from build123d import *

# Parameters (mm, degrees)
PAD_DEPTH = 5


with BuildPart() as part:
    # Sketch → Pad (new body)
    with BuildSketch(Plane.XZ.offset(-65.300003)):
        with BuildLine():
            Line((62.415147, 3.02512), (62.415147, 5.02512))
            Line((62.415147, 5.02512), (55.415147, 5.02512))
            Line((55.415147, 5.02512), (55.415147, 3.02512))
            Line((55.415147, 3.02512), (54.415147, 3.02512))
            add(Edge.make_bspline(
                [(52.415147, 3.02512), (52.415147, 2.62512), (53.415147, 2.62512), (54.415147, 2.62512), (54.415147, 3.02512)],
                knots=[0, 0, 0, 1.570796, 1.570796, 3.141593, 3.141593, 3.141593], degree=2, weights=[1, 0.707107, 1, 0.707107, 1]))
            Line((52.415147, 3.02512), (49.415147, 3.02512))
            add(Edge.make_bspline(
                [(47.415156, 3.02512), (47.417952, 2.625118), (48.417947, 2.625118), (49.417943, 2.625118), (49.415147, 3.02512)],
                knots=[0.003328, 0.003328, 0.003328, 1.574124, 1.574124, 3.144921, 3.144921, 3.144921], degree=2, weights=[1, 0.707107, 1, 0.707107, 1]))
            Line((47.415156, 3.02512), (44.415156, 3.02512))
            add(Edge.make_bspline(
                [(42.415165, 3.02512), (42.417868, 2.625118), (43.417863, 2.625118), (44.417859, 2.625118), (44.415156, 3.02512)],
                knots=[0.003218, 0.003218, 0.003218, 1.574014, 1.574014, 3.14481, 3.14481, 3.14481], degree=2, weights=[1, 0.707107, 1, 0.707107, 1]))
            Line((42.415165, 3.02512), (40.460414, 4.579441))
            ThreePointArc((40.460414, 4.579441), (40.379979, 4.857522), (40.616008, 5.02512))
            Line((40.616008, 5.02512), (53.415147, 5.02512))
            add(Edge.make_bspline(
                [(64.915147, 5.02512), (59.165147, 9.713985), (53.415147, 5.02512)],
                knots=[0.501593, 0.501593, 0.501593, 2.64, 2.64, 2.64], degree=2, weights=[1, 0.480823, 1]))
            Line((64.915147, 5.02512), (66.415147, 5.02512))
            ThreePointArc((66.415147, 5.02512), (68.915147, 2.52512), (66.415147, 0.02512))
            Line((66.415147, 0.02512), (39.399212, 0.02512))
            ThreePointArc((39.399212, 0.02512), (36.86205, 2.118516), (38.435477, 5.007084))
            ThreePointArc((38.435477, 5.007084), (38.564785, 5.022504), (38.684305, 4.970799))
            Line((38.684305, 4.970799), (40.570741, 3.470799))
            ThreePointArc((40.570741, 3.470799), (40.651176, 3.192718), (40.415147, 3.02512))
            Line((40.415147, 3.02512), (39.415147, 3.02512))
            ThreePointArc((39.415147, 3.02512), (38.915147, 2.52512), (39.415147, 2.02512))
            Line((39.415147, 2.02512), (41.784904, 2.02512))
            Line((41.784904, 2.02512), (44.915147, 2.02512))
            add(Edge.make_bspline(
                [(46.915147, 2.02512), (46.915147, 2.42512), (45.915147, 2.42512), (44.915147, 2.42512), (44.915147, 2.02512)],
                knots=[0, 0, 0, 1.570796, 1.570796, 3.141593, 3.141593, 3.141593], degree=2, weights=[1, 0.707107, 1, 0.707107, 1]))
            Line((46.915147, 2.02512), (49.915147, 2.02512))
            add(Edge.make_bspline(
                [(51.915147, 2.02512), (51.915147, 2.42512), (50.915147, 2.42512), (49.915147, 2.42512), (49.915147, 2.02512)],
                knots=[0, 0, 0, 1.570796, 1.570796, 3.141593, 3.141593, 3.141593], degree=2, weights=[1, 0.707107, 1, 0.707107, 1]))
            Line((51.915147, 2.02512), (54.915147, 2.02512))
            add(Edge.make_bspline(
                [(56.915147, 2.02512), (56.915147, 2.42512), (55.915147, 2.42512), (54.915147, 2.42512), (54.915147, 2.02512)],
                knots=[0, 0, 0, 1.570796, 1.570796, 3.141593, 3.141593, 3.141593], degree=2, weights=[1, 0.707107, 1, 0.707107, 1]))
            Line((56.915147, 2.02512), (59.915147, 2.02512))
            add(Edge.make_bspline(
                [(61.915147, 2.02512), (61.915147, 2.42512), (60.915147, 2.42512), (59.915147, 2.42512), (59.915147, 2.02512)],
                knots=[0, 0, 0, 1.570796, 1.570796, 3.141593, 3.141593, 3.141593], degree=2, weights=[1, 0.707107, 1, 0.707107, 1]))
            Line((61.915147, 2.02512), (66.415147, 2.02512))
            ThreePointArc((66.415147, 2.02512), (66.915147, 2.52512), (66.415147, 3.02512))
            Line((66.415147, 3.02512), (64.415147, 3.02512))
            add(Edge.make_bspline(
                [(62.415147, 3.02512), (62.415147, 2.62512), (63.415147, 2.62512), (64.415147, 2.62512), (64.415147, 3.02512)],
                knots=[0, 0, 0, 1.570796, 1.570796, 3.141593, 3.141593, 3.141593], degree=2, weights=[1, 0.707107, 1, 0.707107, 1]))
        make_face()
    extrude(amount=PAD_DEPTH)


solid = part.part
For this review, take the finished solid that the model builds, in its own axes (mm). A direction names the side the tool comes from. Round coordinates to 2 decimals unless told otherwise and drop trailing zeros. Write each loop counter-clockwise with the first axis right and the second up, starting at its lowest first coordinate (ties: lowest second). Pieces come first, ordered by that corner, then holes. Notation, with made-up numbers: (74, 27.5) -> (112, 27.5) arc R33 cw to (112, 55.5) -> close; hole circle Ø6 at (75.25, -11.75). An arc over 180 degrees is marked (long way). Use CSV: the item, a comma, the result in double quotes.
(1) For faces 4 (the face through (47, 63, 5.025)), 5 (the face through (53, 60.3, 3)), 6 (the face through (38.915, 62.835, 2.536)), list the 3-axis set-ups (+Z, -Z, +X, -X, +Y, -Y) from which the entire face can be reached by the end or side of a thin tool; tool diameter is ignored.
Computed values:
face 4,"+Z, -X, +Y, -Y"
face 5,"+Z, -Z, +X, -X, -Y"
face 6,"+Y, -Y"
(2) Draft analysis for pull direction X (two halves, no side actions). For faces 1 (the face through (66, 63, 5.025)), 2 (the face through (68.915, 62.835, 2.58)), 3 (the face through (58, 63, 2.025)), state which applies: +X half, -X half, draft (parallel to the pull), parting line (faces both ways), or undercut.
Computed values:
face 1,"draft"
face 2,"+X half"
face 3,"undercut"
(3) Consider section A-A, the plane x = 66. Give the boundary of the cut face in (y, z), plus the area to 3 significant figures.
Computed values:
outline,"(60.3, 0.03) -> (65.3, 0.03) -> (65.3, 2.03) -> (60.3, 2.03) -> close; (60.3, 3.03) -> (65.3, 3.03) -> (65.3, 5.03) -> (60.3, 5.03) -> close"
area,"20.0 mm²"
(4) Clearance check with flat-ended pins moving along their axes: P1, Ø0.6, axis at y = 63, z = 4.5, coming from the -X side; P2, Ø1.5, axis at x = 53.5, y = 62.5, coming from the +Z side; P3, Ø2.5, axis at x = 42.5, y = 63, coming from the +Z side; P4, Ø2, axis at y = 61, z = 3, coming from the +X side. State where each tip first meets the part, or that it passes through.
Computed values:
P1,"x = 37.36"
P2,"z = 5.56"
P3,"z = 5.03"
P4,"x = 68.92"
(5) Consider section B-B, the plane x = 42. Give the boundary of the cut face in (y, z), plus the area to 3 significant figures.
Computed values:
outline,"(60.3, 0.03) -> (65.3, 0.03) -> (65.3, 2.03) -> (60.3, 2.03) -> close; (60.3, 3.36) -> (65.3, 3.36) -> (65.3, 5.03) -> (60.3, 5.03) -> close"
area,"18.3 mm²"
(6) To check wall thickness, follow L1, parallel to Z at x = 66, y = 63.2; L2, parallel to X at y = 63.45, z = 3.75; L3, parallel to X at y = 61.25, z = 4.75. State the ranges of each line that lie inside material, in increasing order. Write a range as [from, to].
Computed values:
L1,"[0.03, 2.03], [3.03, 5.03]"
L2,"[37.08, 40.22], [41.5, 55.42], [62.42, 68.59]"
L3,"[37.95, 38.96], [40.37, 55.42], [62.42, 67.56]"
